Geometry check sheet. Reference: drawing and pictorial views, mm from the part's lowest x, y, z. A direction names the side the tool comes from. Round coordinates to 2 decimals unless told otherwise and drop trailing zeros. Order: outer loops, then holes, each group sorted by start corner. A loop starts at its lowest first (then second) coordinate and runs counter-clockwise, first axis right, second up.
Q1. Set-up check for the marked faces 4 and 5: record each of +Z, -Z, +X, -X, +Y, -Y from which the full face is reachable in a straight line by a thin tool's end or side.
Q2. Cross-section at C-C on y = 25. Record the cut outline in (x, z).
Q3. Depth check by flat-ended pin: P1, Ø3, axis at y = 8, z = 8, coming from the +X side. Enter the tip coordinate at first touch or a pass-through.
Q4. Cross-section at D-D on x = 58.33. Record the cut outline in (y, z).
Q5. Mould release check, pull along Z, two halves, no side actions. Record for the marked faces 1, 2 and 3: +Z half, -Z half, draft (parallel to the pull), parting line (faces both ways), or undercut.
Q6. Scan lines: probe 1 along Y at (x, z) = (58.33, 3.5); probe 2 along Z at (x, y) = (50.5, 27); probe 3 along X at (y, z) = (4.75, 7.25). Record each from-to range of solid material in increasing order.
Q7. Cross-section at B-B on z = 2. Record the cut outline in (x, y).
Q8. Cross-section at A-A on x = 5. Record the cut outline in (y, z).
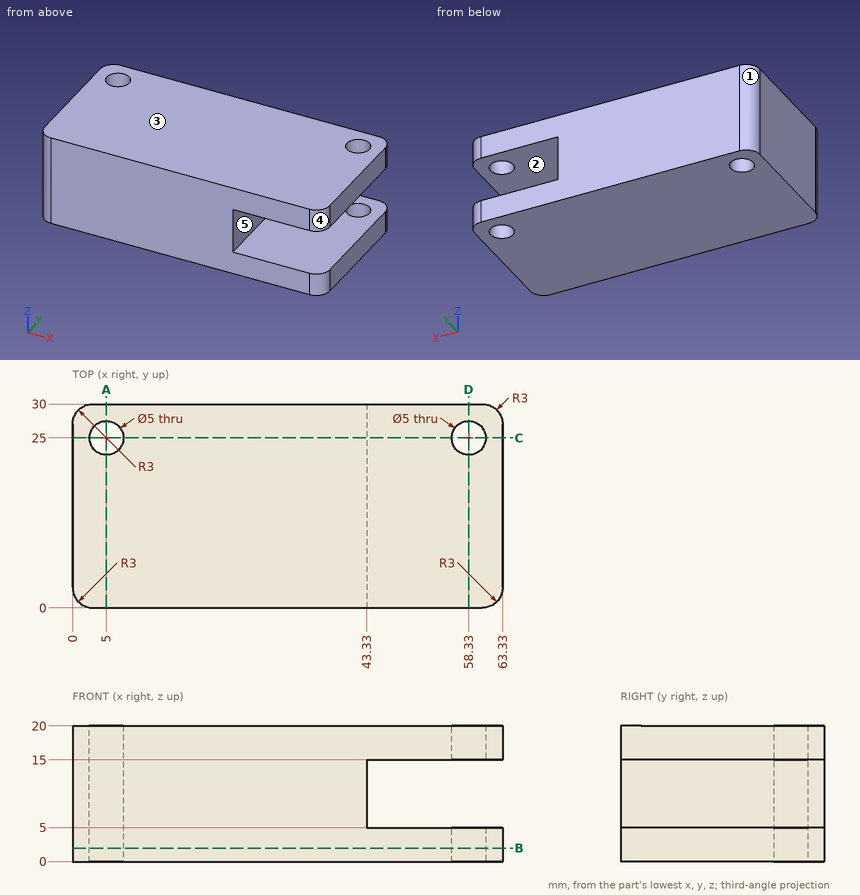
Results found:
1. face 4: +Z, -Z, +X, -Y
1. face 5: +X, +Y, -Y
2. outline: (0, 0) - (2.5, 0) - (2.5, 20) - (0, 20) - close; (7.5, 0) - (55.83, 0) - (55.83, 5) - (43.33, 5) - (43.33, 15) - (55.83, 15) - (55.83, 20) - (7.5, 20) - close; (60.83, 0) - (63.33, 0) - (63.33, 5) - (60.83, 5) - close; (60.83, 15) - (63.33, 15) - (63.33, 20) - (60.83, 20) - close
3. P1: stops at x = 43.33
4. outline: (0, 0) - (22.5, 0) - (22.5, 5) - (0, 5) - close; (0, 15) - (22.5, 15) - (22.5, 20) - (0, 20) - close; (27.5, 0) - (30, 0) - (30, 5) - (27.5, 5) - close; (27.5, 15) - (30, 15) - (30, 20) - (27.5, 20) - close
5. face 1: draft
5. face 2: undercut
5. face 3: +Z half
6. probe 1: y = 0 to 22.5, 27.5 to 30
6. probe 2: z = 0 to 5, 15 to 20
6. probe 3: x = 0 to 43.33
7. outline: (0, 3) arc R3 ccw to (3, 0) - (60.33, 0) arc R3 ccw to (63.33, 3) - (63.33, 27) arc R3 ccw to (60.33, 30) - (3, 30) arc R3 ccw to (0, 27) - close; hole circle Ø5 at (5, 25); hole circle Ø5 at (58.33, 25)
8. outline: (0, 0) - (22.5, 0) - (22.5, 20) - (0, 20) - close; (27.5, 0) - (30, 0) - (30, 20) - (27.5, 20) - close
